The model under review builds one solid part; all positions refer to its coordinate system, in mm. Face numbers are marked on the shaded views. A direction names the side the tool comes from. Round coordinates to 2 decimals unless told otherwise and drop trailing zeros. Loops run counter-clockwise (first coordinate to the right, second up) from the corner with the lowest first, then second, coordinate; pieces in that order, holes last. Notation, with made-up numbers: M 69,44.25 L 117,44.25 A34 ccw 117,81.25 Z; hole C 82.25,-20 d1. An arc over 180 degrees is marked long. Return JSON: item names as keys, results as strings. Group by question number.
Q1. Consider section C-C (y = 37.5). State the section outline as (x, z) points, and give its area (3 significant figures).
Q2. Draft analysis for pull direction X (two halves, no side actions). For the marked faces 4, 5, 6 and 7, state which applies: pulls with the +X half, pulls with the -X half, needs draft (parallel to the pull), parting line crosses it, or undercut.
Q3. To check wall thickness, follow line 1 along Y through (x, z) = (0, 14.5); line 2 along Y through (x, z) = (-12, 5.5); line 3 along X through (y, z) = (-33, 27). State the ranges of each line that lie inside material, in increasing order.
Q4. Consider section B-B (x = -2). Count the separate pieces of the cut face and the enclosed holes in it, and give its area (3 significant figures).
Q5. Clearance check with flat-ended pins moving along their axes: pin 1 Ø4 at (x, y) = (18, 28) entering from -Z; pin 2 Ø0.5 at (x, z) = (-16, 7) entering from -Y; pin 3 Ø18.5 at (x, y) = (5, 36) entering from +Z; pin 4 Ø2 at (y, z) = (39.5, 7) entering from +X. State where each tip first meets the part, or that it passes through.
Q6. Consider section D-D (y = -5). State the section outline as (x, z) points, and give its area (3 significant figures).
Q7. For the marked faces 1, 2 and 3, list the 3-axis set-ups (+Z, -Z, +X, -X, +Y, -Y) from which the entire face can be reached by the end or side of a thin tool; tool diameter is ignored.
Q8. Consider section A-A (z = 23.5). State the section outline as (x, y) points.
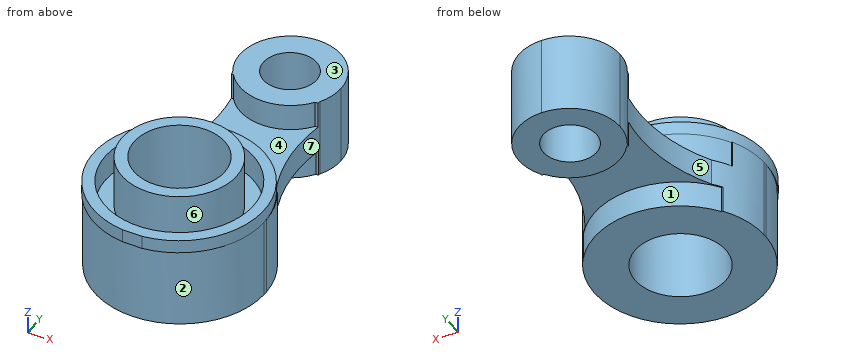
from build123d import *

# Parameters (mm, degrees)
ESQUISSE1_W              = 64
ESQUISSE1_H              = 126
BOSS_EXTRU_1_DEPTH       = 45
ESQUISSE2_W              = 74.759642061
ESQUISSE2_H              = 139.382383503
ESQUISSE2_R              = 32
ENL_V_MAT_EXTRU_2_DEPTH  = 15
ESQUISSE3_R              = 27.5
ENL_V_MAT_EXTRU_5_DEPTH  = 10
ESQUISSE5_R              = 27.775
ESQUISSE5_R_2            = 21.5
ENL_V_MAT_EXTRU_7_DEPTH  = 20
ESQUISSE6_R              = 17
ENL_V_MAT_EXTRU_8_DEPTH  = 84.773504165
ESQUISSE7_R              = 10
ENL_V_MAT_EXTRU_9_DEPTH  = 77.765877836
ESQUISSE8_W              = 86.397385067
ESQUISSE8_H              = 136.429769075
ENL_V_MAT_EXTRU_11_DEPTH = 77.765877836
ENL_V_MAT_EXTRU_12_DEPTH = 10
ENL_V_MAT_EXTRU_13_DEPTH = 10


with BuildPart() as part:
    # Esquisse1 → Boss.-Extru.1 (new body)
    with BuildSketch(Plane.XY):
        Rectangle(ESQUISSE1_W, ESQUISSE1_H)
    extrude(amount=BOSS_EXTRU_1_DEPTH)

    # Esquisse2 → Enlèv. mat.-Extru.2 (cut)
    with BuildSketch(Plane.XY.offset(45)):
        with Locations((-0.51685586, -5.363099381)):
            Rectangle(ESQUISSE2_W, ESQUISSE2_H)
        with Locations((0, -31.212195959)):
            Circle(ESQUISSE2_R, mode=Mode.SUBTRACT)
    extrude(amount=-ENL_V_MAT_EXTRU_2_DEPTH, mode=Mode.SUBTRACT)

    # Esquisse3 → Enlèv. mat.-Extru.5 (cut)
    with BuildSketch(Plane.XY.offset(45)):
        with BuildLine():
            Line((-3.679064313, -63), (3.679064313, -63))
            ThreePointArc((3.679064313, -63), (0, 0.787804041), (-3.679064313, -63))
        make_face()
        with Locations((0, -31.212195959)):
            Circle(ESQUISSE3_R, mode=Mode.SUBTRACT)
    extrude(amount=-ENL_V_MAT_EXTRU_5_DEPTH, mode=Mode.SUBTRACT)

    # Esquisse5 → Enlèv. mat.-Extru.7 (cut)
    with BuildSketch(Plane.XY.offset(45)):
        with Locations((0, -31)):
            Circle(ESQUISSE5_R)
        with Locations((0, -31)):
            Circle(ESQUISSE5_R_2, mode=Mode.SUBTRACT)
    extrude(amount=-ENL_V_MAT_EXTRU_7_DEPTH, mode=Mode.SUBTRACT)

    # Esquisse6 → Enlèv. mat.-Extru.8 (cut, through all)
    with BuildSketch(Plane.XY.offset(45)):
        with Locations((0, -30.914318574)):
            Circle(ESQUISSE6_R)
    extrude(amount=-ENL_V_MAT_EXTRU_8_DEPTH, mode=Mode.SUBTRACT)

    # Esquisse7 → Enlèv. mat.-Extru.9 (cut, through all)
    with BuildSketch(Plane.XY.offset(30)):
        with Locations((0, 44)):
            Circle(ESQUISSE7_R)
    extrude(amount=-ENL_V_MAT_EXTRU_9_DEPTH, mode=Mode.SUBTRACT)

    # Esquisse8 → Enlèv. mat.-Extru.11 (cut, through all)
    with BuildSketch(Plane.XY.offset(30)):
        with Locations((-1.464362458, -2.806694712)):
            Rectangle(ESQUISSE8_W, ESQUISSE8_H)
        with BuildLine():
            Line((-32, 63), (0.202169279, 63))
            Line((0.202169279, 63), (32, 63))
            Line((32, 63), (32, -29.80290649))
            ThreePointArc((32, -29.80290649), (32.005817879, -30.155207508), (32.00775725, -30.507551224))
            ThreePointArc((32.00775725, -30.507551224), (32.005817879, -30.85989494), (32, -31.212195959))
            ThreePointArc((32, -31.212195959), (0, -62.515308475), (-32, -31.212195959))
            ThreePointArc((-32, -31.212195959), (-32.00775725, -30.507551224), (-32, -29.80290649))
            Line((-32, -29.80290649), (-32, 63))
        make_face(mode=Mode.SUBTRACT)
        with BuildLine():
            ThreePointArc((0.202169279, 63), (13.63719816, 57.435028864), (19.202169338, 44))
            ThreePointArc((19.202169338, 44), (18.538621544, 39.022599022), (16.594325075, 34.392855247))
            ThreePointArc((16.594325075, 34.392855247), (16.343681733, 11.978736432), (23.83747578, -9.147043911))
            ThreePointArc((23.83747578, -9.147043911), (29.76780291, -18.744284921), (32, -29.80290649))
            Line((32, -29.80290649), (32, 63))
            Line((32, 63), (0.202169279, 63))
        make_face()
        with BuildLine():
            ThreePointArc((-18.797830662, 44), (-13.232859525, 57.435028822), (0.202169279, 63))
            Line((0.202169279, 63), (-32, 63))
            Line((-32, 63), (-32, -29.80290649))
            ThreePointArc((-32, -29.80290649), (-29.74748685, -18.693002977), (-23.763712379, -9.065011772))
            ThreePointArc((-23.763712379, -9.065011772), (-16.134588528, 12.08350842), (-16.289948146, 34.565485657))
            ThreePointArc((-16.289948146, 34.565485657), (-18.160159384, 39.118925948), (-18.797830662, 44))
        make_face()
    extrude(amount=-ENL_V_MAT_EXTRU_11_DEPTH, mode=Mode.SUBTRACT)

    # Esquisse10 → Enlèv. mat.-Extru.12 (cut)
    with BuildSketch(Plane.XY.offset(30)):
        with BuildLine():
            Line((-15.358096219, 33.354922672), (-16.07732259, 33.354922672))
            ThreePointArc((-16.07732259, 33.354922672), (-16.24125544, 11.478282043), (-23.763712379, -9.065011772))
            ThreePointArc((-23.763712379, -9.065011772), (-26.135325713, -12.029421609), (-28.139276, -15.253775612))
            Line((-28.139276, -15.253775612), (-27.736777391, -15.253775612))
            ThreePointArc((-27.736777391, -15.253775612), (0, 0.787804041), (27.736777391, -15.253775612))
            Line((27.736777391, -15.253775612), (28.139276, -15.253775612))
            ThreePointArc((28.139276, -15.253775612), (26.167130611, -12.074488543), (23.83747578, -9.147043911))
            ThreePointArc((23.83747578, -9.147043911), (16.432370726, 11.458852589), (16.406556938, 33.354922672))
            Line((16.406556938, 33.354922672), (15.358096219, 33.354922672))
            ThreePointArc((15.358096219, 33.354922672), (0, 25.541024787), (-15.358096219, 33.354922672))
        make_face()
    extrude(amount=-ENL_V_MAT_EXTRU_12_DEPTH, mode=Mode.SUBTRACT)

    # Esquisse11 → Enlèv. mat.-Extru.13 (cut)
    with BuildSketch(Plane(origin=(0, 0, 0), x_dir=(-1, 0, 0), z_dir=(0, 0, -1))):
        with BuildLine():
            Line((-15.504189616, 33.558306347), (-16.441959806, 33.558306347))
            ThreePointArc((-16.441959806, 33.558306347), (-16.41467553, 11.560545546), (-23.83747578, -9.147043911))
            ThreePointArc((-23.83747578, -9.147043911), (-25.093902529, -10.63816321), (-26.257202417, -12.20302049))
            Line((-26.257202417, -12.20302049), (-26.162723497, -12.20302049))
            ThreePointArc((-26.162723497, -12.20302049), (-0.203383675, 1.085681426), (25.755956147, -12.20302049))
            Line((25.755956147, -12.20302049), (26.257202417, -12.20302049))
            ThreePointArc((26.257202417, -12.20302049), (25.059623979, -10.594947923), (23.763712379, -9.065011772))
            ThreePointArc((23.763712379, -9.065011772), (16.222953758, 11.579751881), (16.111372133, 33.558306347))
            Line((16.111372133, 33.558306347), (15.504189616, 33.558306347))
            ThreePointArc((15.504189616, 33.558306347), (0, 25.541024787), (-15.504189616, 33.558306347))
        make_face()
    extrude(amount=-ENL_V_MAT_EXTRU_13_DEPTH, mode=Mode.SUBTRACT)


solid = part.part
Values:
{
 "1": {"outline": "M -17.65,0 L -7.6,0 L -7.6,30 L -17.65,30 Z; M 7.6,0 L 18.06,0 L 18.06,30 L 7.6,30 Z", "area": "615 mm2"},
 "2": {"face 4": "needs draft", "face 5": "pulls with the -X half", "face 6": "undercut", "face 7": "pulls with the +X half"},
 "3": {"line 1": "y = -62.52 to -47.91, -13.91 to 34, 54 to 63", "line 2": "y = -60.18 to -42.96, -18.87 to -1.33, 29.81 to 58.56", "line 3": "x = -31.91 to -27.7, -21.41 to -16.87, 16.87 to 21.41, 27.7 to 31.91"},
 "4": {"separate pieces": "3", "enclosed holes": "0", "area": "1,780 mm2"},
 "5": {"pin 1": "passes through", "pin 2": "stops at y = -58.37", "pin 3": "stops at z = 30", "pin 4": "stops at x = 18.88"},
 "6": {"outline": "M -21.61,10 L -18.57,10 L -18.57,0 L 18.98,0 L 18.98,10 L 21.68,10 L 21.68,20 L 18.36,20 L 18.36,35 L 9.77,35 L 9.77,25 L -9.77,25 L -9.77,35 L -18.36,35 L -18.36,20 L -21.61,20 Z", "area": "1,160 mm2"},
 "7": {"face 1": "-Z", "face 2": "-Z, -Y", "face 3": "+Z, +X, -X, +Y"},
 "8": {"outline": "M -32,-31.21 A32.01 ccw 32,-31.21 L 32,-29.8 A32.01 ccw 28.14,-15.25 L 27.74,-15.25 A32 ccw -27.74,-15.25 L -28.14,-15.25 A32.01 ccw -32,-29.8 Z; M -16.29,34.57 A64 cw -16.08,33.35 L -15.36,33.35 A19 ccw 15.36,33.35 L 16.41,33.35 A64 cw 16.59,34.39 A19 ccw long Z; hole C 0,-30.91 d34; hole C 0,44 d20"}
}
